Geometry check sheet. Reference: the model listing, model coordinates, mm. A direction names the side the tool comes from. Round coordinates to 2 decimals unless told otherwise and drop trailing zeros. Order: outer loops, then holes, each group sorted by start corner. A loop starts at its lowest first (then second) coordinate and runs counter-clockwise, first axis right, second up.
```python
from build123d import *

# Parameters (mm, degrees)
F1_W         = 27
F1_H         = 43.8
F1_R         = 1.5
F1_H_2       = 7
F2_DEPTH     = 34
F3_R         = 1.75
F4_DEPTH     = 57.801
F5_W         = 43.8
F5_H         = 26
F6_DEPTH     = 27.001
F7_DEPTH     = 10
F8_DEPTH     = 10
F9_T4_DEPTH  = 26.8933659759
F9_S5_R      = 1.75
F9_T6_DEPTH  = 15
F9_T10_DEPTH = 26.8933659759
F9_S11_R     = 1.75
F9_T12_DEPTH = 15
F9_T16_DEPTH = 26.8933659759
F9_S17_R     = 1.75
F9_T18_DEPTH = 15
F9_T22_DEPTH = 26.8933659759
F9_S23_R     = 1.75
F9_T24_DEPTH = 15
F12_DEPTH    = 2.5
F14_DEPTH    = 2
F15_SIZE     = 10
F16_R        = 1.75
F17_DEPTH    = 51.5
F18_R        = 3
F19_DEPTH    = 4
F21_DEPTH    = 2.5
F22_DEPTH    = 47
F24_DEPTH    = 2.5
F25_R        = 1.25
F26_DEPTH    = 3
F27_R        = 2
F28_T1_DEPTH = 1
F28_T3_DEPTH = 3
F28_T8_ANGLE = 161.6484946187


# Not quite as in the source:
# - a fillet or chamfer that OpenCascade refuses, or shapes differently, is made with other operations: its cross-section is extruded or revolved along the edge and cut away or added


with BuildPart() as f2:
    # F1 (on Top) → F2 (new body)
    with BuildSketch(Plane.XY):
        Rectangle(F1_W, F1_H)
        with Locations((-10, -10)):
            Circle(F1_R, mode=Mode.SUBTRACT)
        with Locations((10, -10)):
            Circle(F1_R, mode=Mode.SUBTRACT)
        with Locations((-10, 10)):
            Circle(F1_R, mode=Mode.SUBTRACT)
        with Locations((10, 10)):
            Circle(F1_R, mode=Mode.SUBTRACT)
        with Locations((0, 25.4)):
            Rectangle(F1_W, F1_H_2)
        with Locations((0, -25.4)):
            Rectangle(F1_W, F1_H_2)
    extrude(amount=F2_DEPTH)

    # F3 (on face) → F4 (cut, through all)
    with BuildSketch(Plane(origin=(0, 28.9, 0), x_dir=(-1, 0, 0), z_dir=(0, 1, 0))):
        with Locations((0, 27.395)):
            Circle(F3_R)
        with Locations((0, 8)):
            Circle(F3_R)
    extrude(amount=-F4_DEPTH, mode=Mode.SUBTRACT)

    # F5 (on face) → F6 (cut, through all)
    with BuildSketch(Plane(origin=(-13.5, 0, 0), x_dir=(0, -1, 0), z_dir=(-1, 0, 0))):
        with Locations((0, 21)):
            Rectangle(F5_W, F5_H)
    extrude(amount=-F6_DEPTH, mode=Mode.SUBTRACT)

    # F7 (add): a face of the model
    f7_faces = [f2.faces().sort_by_distance(p)[0] for p in [
        (-13.5, 0, 0.6705848194),
    ]]
    extrude(f7_faces, amount=F7_DEPTH)

    # F8 (add): a face of the model
    f8_faces = [f2.faces().sort_by_distance(p)[0] for p in [
        (13.5, 0, 0.6705848194),
    ]]
    extrude(f8_faces, amount=F8_DEPTH)

    # F9: chamfer of 2 on 4 edges, made by hand


with BuildPart() as f9_tool2:
    # F9_s3 → F9_t4 (new body)
    with BuildSketch(Plane.YZ.offset(3.3933659759)):
        Polygon((-21.9, 10), (-19.9, 8), (-21.9, 8), align=None)
    extrude(amount=-F9_T4_DEPTH)

    # F9_s5 → F9_t6 (cut, symmetric)
    with BuildSketch(Plane.XZ.offset(20.9)):
        with Locations((0, 8)):
            Circle(F9_S5_R)
    extrude(amount=F9_T6_DEPTH, both=True, mode=Mode.SUBTRACT)


with BuildPart() as f2_1:
    add(f2.part)

    # F9_t1: union F9_tool2
    add(f9_tool2.part)


with BuildPart() as f9_tool8:
    # F9_s9 → F9_t10 (new body)
    with BuildSketch(Plane.YZ.offset(-23.5)):
        Polygon((21.9, 10), (19.9, 8), (21.9, 8), align=None)
    extrude(amount=F9_T10_DEPTH)

    # F9_s11 → F9_t12 (cut, symmetric)
    with BuildSketch(Plane.XZ.offset(-20.9)):
        with Locations((0, 8)):
            Circle(F9_S11_R)
    extrude(amount=F9_T12_DEPTH, both=True, mode=Mode.SUBTRACT)


with BuildPart() as f2_2:
    add(f2_1.part)

    # F9_t7: union F9_tool8
    add(f9_tool8.part)


with BuildPart() as f9_tool14:
    # F9_s15 → F9_t16 (new body)
    with BuildSketch(Plane.YZ.offset(-3.3933659759)):
        Polygon((21.9, 10), (19.9, 8), (21.9, 8), align=None)
    extrude(amount=F9_T16_DEPTH)

    # F9_s17 → F9_t18 (cut, symmetric)
    with BuildSketch(Plane.XZ.offset(-20.9)):
        with Locations((0, 8)):
            Circle(F9_S17_R)
    extrude(amount=F9_T18_DEPTH, both=True, mode=Mode.SUBTRACT)


with BuildPart() as f2_3:
    add(f2_2.part)

    # F9_t13: union F9_tool14
    add(f9_tool14.part)


with BuildPart() as f9_tool20:
    # F9_s21 → F9_t22 (new body)
    with BuildSketch(Plane.YZ.offset(23.5)):
        Polygon((-19.9, 8), (-21.9, 10), (-21.9, 8), align=None)
    extrude(amount=-F9_T22_DEPTH)

    # F9_s23 → F9_t24 (cut, symmetric)
    with BuildSketch(Plane.XZ.offset(20.9)):
        with Locations((0, 8)):
            Circle(F9_S23_R)
    extrude(amount=F9_T24_DEPTH, both=True, mode=Mode.SUBTRACT)


with BuildPart() as f2_4:
    add(f2_3.part)

    # F9_t19: union F9_tool20
    add(f9_tool20.part)

    # F11 (on face) → F12 (join)
    with BuildSketch(Plane(origin=(-23.5, 0, 0), x_dir=(0, -1, 0), z_dir=(-1, 0, 0))):
        Polygon((-28.9, 50), (-28.9, 34), (-28.9, 0), (28.9, 0), (28.9, 50), align=None)
    extrude(amount=F12_DEPTH)

    # F13 (on face) → F14 (join)
    with BuildSketch(Plane.YZ.offset(23.5)):
        Polygon((-28.9, 34), (-28.9, 28), (-28.9, 0), (28.9, 0), (28.9, 28), (28.9, 34), (28.9, 50), (-28.9, 50), align=None)
    extrude(amount=F14_DEPTH)

    # F15
    f15_edges = [f2_4.edges().sort_by_distance(p)[0] for p in [
        (-24.75, 28.9, 50),
        (-24.75, -28.9, 50),
        (24.5, -28.9, 50),
        (24.5, 28.9, 50),
    ]]
    chamfer(f15_edges, length=F15_SIZE)

    # F16 (on face) → F17 (cut, through all)
    with BuildSketch(Plane.YZ.offset(25.5)):
        with BuildLine():
            Line((-12, 50), (-12, 29.15))
            ThreePointArc((-12, 29.15), (0, 17.15), (12, 29.15))
            Line((12, 29.15), (12, 50))
            Line((12, 50), (-12, 50))
        make_face()
        with Locations((-15.5, 44.65)):
            Circle(F16_R)
        with Locations((15.5, 44.65)):
            Circle(F16_R)
        with Locations((15.5, 13.65)):
            Circle(F16_R)
        with Locations((-15.5, 13.65)):
            Circle(F16_R)
    extrude(amount=-F17_DEPTH, mode=Mode.SUBTRACT)

    # F18 (on face) → F19 (cut)
    with BuildSketch(Plane.XY.offset(8)):
        with Locations((10, -10)):
            Circle(F18_R)
        with Locations((10, 10)):
            Circle(F18_R)
        with Locations((-10, -10)):
            Circle(F18_R)
        with Locations((-10, 10)):
            Circle(F18_R)
    extrude(amount=-F19_DEPTH, mode=Mode.SUBTRACT)

    # F20 (on face) → F21 (cut)
    with BuildSketch(Plane.XZ.offset(-21.9)):
        Polygon((2.75, 25.8072867597), (2.75, 28.9827132403), (0, 30.5704264805), (-2.75, 28.9827132403), (-2.75, 25.8072867597), (0, 24.2195735195), align=None)
        Polygon((2.75, 6.3760742294), (2.75, 9.55150071), (0, 11.1392139502), (-2.75, 9.55150071), (-2.75, 6.3760742294), (0, 4.7883609892), align=None)
    extrude(amount=-F21_DEPTH, mode=Mode.SUBTRACT)

    # F20 (on face) → F22 (cut)
    with BuildSketch(Plane.XZ.offset(-21.9)):
        Polygon((2.75, 6.3760742294), (2.75, 9.55150071), (1.9731764425, 10), (-1.9731764425, 10), (-2.75, 9.55150071), (-2.75, 6.3760742294), (0, 4.7883609892), align=None)
    extrude(amount=F22_DEPTH, mode=Mode.SUBTRACT)

    # F23 (on face) → F24 (cut)
    with BuildSketch(Plane(origin=(0, -21.9, 0), x_dir=(-1, 0, 0), z_dir=(0, 1, 0))):
        Polygon((2.75, 25.8072867597), (2.75, 28.9827132403), (0, 30.5704264805), (-2.75, 28.9827132403), (-2.75, 25.8072867597), (0, 24.2195735195), align=None)
        Polygon((2.75, 6.4122867597), (2.75, 9.5877132403), (0, 11.1754264805), (-2.75, 9.5877132403), (-2.75, 6.4122867597), (0, 4.8245735195), align=None)
    extrude(amount=-F24_DEPTH, mode=Mode.SUBTRACT)

    # F25 (on face) → F26 (join)
    with BuildSketch(Plane(origin=(-26, 0, 0), x_dir=(0, -1, 0), z_dir=(-1, 0, 0))):
        Polygon((28.9, 2), (28.9, 0), (40.9, 0), (40.9, 12.8), (28.9, 12.8), (28.9, 4), (31.9, 4), (31.9, 2), align=None)
        with Locations((35.9, 3.15)):
            Circle(F25_R, mode=Mode.SUBTRACT)
        with Locations((35.9, 9.65)):
            Circle(F25_R, mode=Mode.SUBTRACT)
    extrude(amount=-F26_DEPTH)

    # F27
    f27_edges = [f2_4.edges().sort_by_distance(p)[0] for p in [
        (-24.5, -28.9, 12.8),
        (23.5, -25.4, 34),
        (-23.5, -25.4, 34),
        (-23.5, 25.4, 34),
        (23.5, 25.4, 34),
        (-23, -28.9, 8.4),
        (-23, -28.9, 1),
        (24.5, 28.9, 40),
        (-24.75, 28.9, 40),
        (-24.75, 18.9, 50),
        (-24.75, -12, 50),
        (-24.75, 12, 50),
        (-24.75, -18.9, 50),
        (24.5, -12, 50),
        (24.5, 12, 50),
        (24.5, -18.9, 50),
        (24.5, -28.9, 40),
        (-24.75, -28.9, 40),
        (24.5, 18.9, 50),
    ]]
    fillet(f27_edges, radius=F27_R)

    # F28: fillet of radius 1 on 3 edges, made by hand

    # F28_s2 → F28_t1 (cut)
    with BuildSketch(Plane.XZ.offset(30.9)):
        with BuildLine():
            ThreePointArc((-24, 2), (-23.2928932188, 1.7071067812), (-23, 1))
            Line((-23, 1), (-23, 2))
            Line((-23, 2), (-24, 2))
        make_face()
    extrude(amount=F28_T1_DEPTH, mode=Mode.SUBTRACT)

    # F28_s4 → F28_t3 (cut)
    with BuildSketch(Plane.XZ.offset(28.9)):
        with BuildLine():
            ThreePointArc((-26, 1), (-25.7071067812, 1.7071067812), (-25, 2))
            Line((-25, 2), (-26, 2))
            Line((-26, 2), (-26, 1))
        make_face()
    extrude(amount=F28_T3_DEPTH, mode=Mode.SUBTRACT)


with BuildPart() as f28_tool6:
    # F28_s7 → F28_t8 (revolve)
    with BuildSketch(Plane(origin=(7.1522739521, -21.561442082, 0), x_dir=(0, 0, 1), z_dir=(0.3148458041, -0.9491428342, 0))):
        with BuildLine():
            ThreePointArc((2, 26.6607348638), (1.7071067812, 27.367841645), (1, 27.6607348638))
            Line((1, 27.6607348638), (2, 27.6607348638))
            Line((2, 27.6607348638), (2, 26.6607348638))
        make_face()
    revolve(axis=Axis((-21, -30.9, 2), (0, 0, 1)), revolution_arc=F28_T8_ANGLE)

    split(bisect_by=Plane.XZ.offset(28.9), keep=Keep.TOP)


with BuildPart() as f2_5:
    add(f2_4.part)

    # F28_t5: cut F28_tool6
    add(f28_tool6.part, mode=Mode.SUBTRACT)


solid = f2_5.part
```
(1) Set-up check for faces 4 (the flat face through (-8.7, -11.3, 4)), 5 (the flat face through (-24.5, -30.4, 2)), 6 (the cylindrical face through (22.9, -25.35, 34.57)), 7 (the flat face through (2.75, 0, 7.6)): record each of +Z, -Z, +X, -X, +Y, -Y from which the full face is reachable in a straight line by a thin tool's end or side.
Returned:
face 4: +Z
face 5: +X, -X
face 6: +Z, +Y, -Y
face 7: none
(2) Depth check by flat-ended pin: P1, Ø3.5, axis at x = -10, y = -10, coming from the +Z side; P2, Ø6.5, axis at x = 10, y = -9.5, coming from the +Z side; P3, Ø5, axis at x = 1.5, z = 32.5, coming from the -Y side. Enter the tip coordinate at first touch or a pass-through.
Returned:
P1: stops at z = 4
P2: stops at z = 8
P3: stops at y = -28.9
(3) Sectioned sample at B-B, the plane y = -15.5. Give the number of separate pieces and of enclosed holes in the cut face, and give its area (3 significant figures).
Returned:
separate pieces: 5
enclosed holes: 0
area: 556 mm2
(4) Sectioned sample at C-C, the plane x = -10. Record the cut outline in (y, z).
Returned:
outline: (-28.9, 0) - (-11.5, 0) - (-11.5, 4) - (-13, 4) - (-13, 8) - (-19.9, 8) - (-21.9, 10) - (-21.9, 34) - (-28.9, 34) - close; (-8.5, 0) - (8.5, 0) - (8.5, 4) - (7, 4) - (7, 8) - (-7, 8) - (-7, 4) - (-8.5, 4) - close; (11.5, 0) - (28.9, 0) - (28.9, 34) - (21.9, 34) - (21.9, 10) - (19.9, 8) - (13, 8) - (13, 4) - (11.5, 4) - close
(5) Sectioned sample at D-D, the plane z = 13.65. Record the cut outline in (x, y).
Returned:
outline: (-26, -29.26) - (-22.15, -29.26) arc R2 cw to (-21, -28.9) - (25.5, -28.9) - (25.5, -17.25) - (23.5, -17.25) - (23.5, -21.9) - (-23.5, -21.9) - (-23.5, -17.25) - (-26, -17.25) - close; (-26, -13.75) - (-23.5, -13.75) - (-23.5, 13.75) - (-26, 13.75) - close; (-26, 17.25) - (-23.5, 17.25) - (-23.5, 21.9) - (23.5, 21.9) - (23.5, 17.25) - (25.5, 17.25) - (25.5, 28.9) - (-26, 28.9) - close; (23.5, -13.75) - (25.5, -13.75) - (25.5, 13.75) - (23.5, 13.75) - close
(6) Draft check along Z on faces 1 (the flat face through (-1.356, -23.132, 25.002)), 2 (the flat face through (23.5, 12.4, 29.3)), 3 (the flat face through (12.6, 20.9, 9)). Enter one of: released by +Z, released by -Z, zero draft, split by the parting line, or undercut.
Returned:
face 1: undercut
face 2: zero draft
face 3: released by +Z
(7) Material ranges on line 1 (Y direction, x = 10, z = 5.7); line 2 (Y direction, x = -24, z = 3); line 3 (Z direction, x = -24.3, y = -35.9), recorded low to high.
Returned:
line 1: y = -28.9 to -13, -7 to 7, 13 to 28.9
line 2: y = -40.9 to -37.14, -34.66 to -31.9, -28.9 to 28.9
line 3: z = 0 to 1.9, 4.4 to 8.4, 10.9 to 12.8
(8) Sectioned sample at A-A, the plane y = -35.9. Record the cut outline in (x, z), and give its area (3 significant figures).
Returned:
outline: (-26, 0) - (-23, 0) - (-23, 1.9) - (-26, 1.9) - close; (-26, 4.4) - (-23, 4.4) - (-23, 8.4) - (-26, 8.4) - close; (-26, 10.9) - (-23, 10.9) - (-23, 12.8) - (-26, 12.8) - close
area: 23.4 mm2
